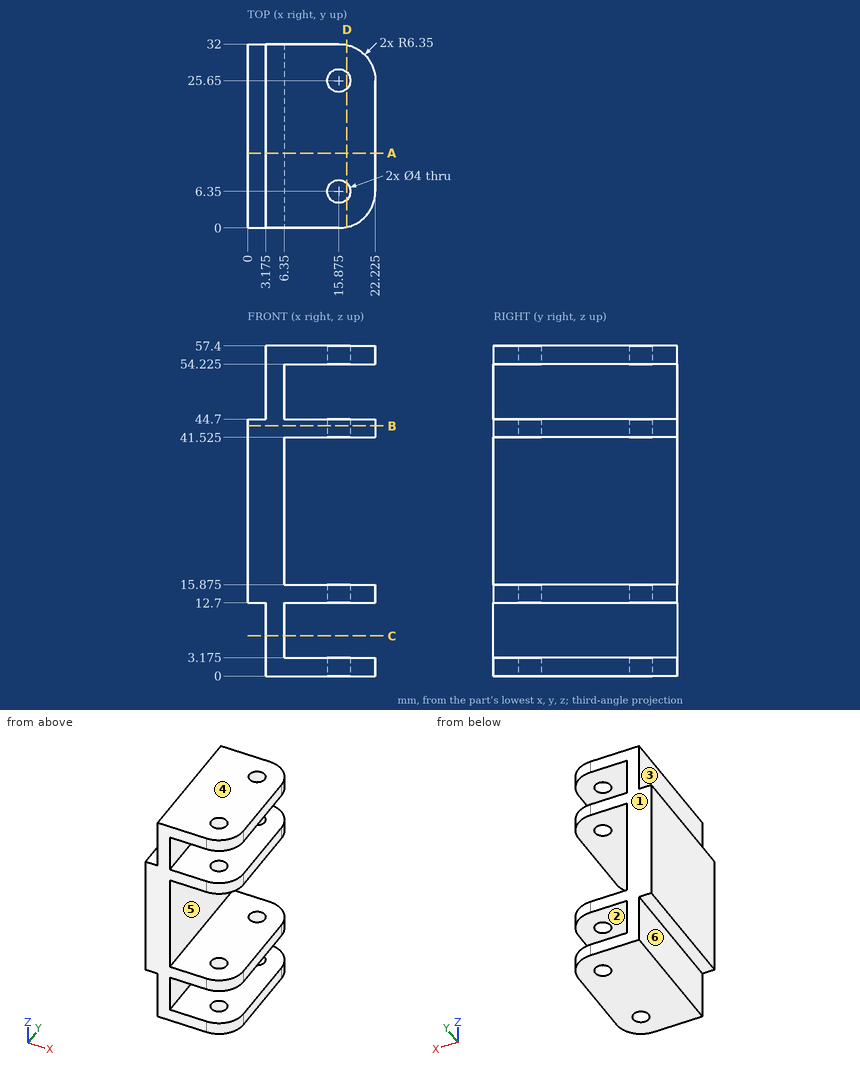
Study the drawing (mm; zero at the part's minimum x, y, z) and answer. A direction names the side the tool comes from. Coordinates: 2 decimals unless noted, no trailing zeros. Write each loop counter-clockwise with the first axis right and the second up, starting at its lowest first coordinate (ties: lowest second). Pieces come first, ordered by that corner, then holes. Notation, with made-up numbers: (11, 46.25) - (62, 46.25) arc R23 ccw to (62, 72.25) - close; hole circle Ø3 at (80.5, 52.5). An arc over 180 degrees is marked (long way). One line per item, written item: value.
1) For a pull along Z with two mould halves and no side action, classify the marked faces 4, 5 and 6 as pulls with the +Z half, pulls with the -Z half, needs draft (parallel to the pull), parting line crosses it, or undercut.
Geometry check:
face 4: pulls with the +Z half
face 5: undercut
face 6: needs draft
2) A tool of negligible diameter and unlimited length cuts with its end or side. For the marked faces 1, 2 and 3, from which of +Z, -Z, +X, -X, +Y, -Y can it reach the whole face along a straight path? Write none if from no direction.
Geometry check:
face 1: +Z, -Z, +X, -X, +Y
face 2: +X, +Y, -Y
face 3: +Z, -X, +Y, -Y
3) Each of these flat-tipped pins is pushed along its axis until it touches: pin 1 Ø3 at (y, z) = (25, 22) entering from +X; pin 2 Ø6 at (y, z) = (11, 7.5) entering from -X (3 decimals); pin 3 Ø1.6 at (x, y) = (1, 12.5) entering from +Z. Where does it stop, or does it pass through?
Geometry check:
pin 1: stops at x = 6.35
pin 2: stops at x = 3.175
pin 3: stops at z = 44.7
4) Consider line 1 along Z through (x, y) = (20.25, 27) (3 decimals); line 2 along X through (y, z) = (25.65, 43.9) (3 decimals); line 3 along X through (y, z) = (25.65, 55.75) (3 decimals). Determine where each line is inside the solid, lowest interval first. Write a range as from..to.
Geometry check:
line 1: z = 0..3.175, 12.7..15.875, 41.525..44.7, 54.225..57.4
line 2: x = 0..13.875, 17.875..22.225
line 3: x = 3.175..13.875, 17.875..22.225
5) Find section B-B (z = 43.5). Give the vertices of the cut face in (x, y) (3 decimals).
Geometry check:
outline: (0, 0) - (15.875, 0) arc R6.35 ccw to (22.225, 6.35) - (22.225, 25.65) arc R6.35 ccw to (15.875, 32) - (0, 32) - close; hole circle Ø4 at (15.875, 6.35); hole circle Ø4 at (15.875, 25.65)
6) Find section A-A (y = 13). Give the vertices of the cut face in (x, z) (3 decimals), and give its area (3 significant figures).
Geometry check:
outline: (0, 12.7) - (3.175, 12.7) - (3.175, 0) - (22.225, 0) - (22.225, 3.175) - (6.35, 3.175) - (6.35, 12.7) - (22.225, 12.7) - (22.225, 15.875) - (6.35, 15.875) - (6.35, 41.525) - (22.225, 41.525) - (22.225, 44.7) - (6.35, 44.7) - (6.35, 54.225) - (22.225, 54.225) - (22.225, 57.4) - (3.175, 57.4) - (3.175, 44.7) - (0, 44.7) - close
area: 485 mm2
7) Find section D-D (x = 17.25). Count the separate pieces of the cut face and the enclosed holes in it, and give its area (3 significant figures).
Geometry check:
separate pieces: 12
enclosed holes: 0
area: 329 mm2
8) Find section C-C (z = 7). Give the vertices of the cut face in (x, y) (3 decimals).
Geometry check:
outline: (3.175, 0) - (6.35, 0) - (6.35, 32) - (3.175, 32) - close
